```python
from build123d import *

# Parameters (mm, degrees)
SKETCH1_R           = 50.8
BOSS_EXTRUDE1_DEPTH = 203.2
SKETCH2_W           = 63.5
SKETCH2_H           = 79.31147458
BOSS_EXTRUDE2_DEPTH = 63.5
SKETCH3_W           = 25.4
SKETCH3_H           = 79.31147458
CUT_EXTRUDE1_DEPTH  = 63.5
FILLET1_R           = 25.4
SKETCH4_R           = 31.75
CUT_EXTRUDE2_DEPTH  = 63.5
SKETCH6_W           = 101.6
SKETCH6_H           = 101.6
BOSS_EXTRUDE3_DEPTH = 254
SKETCH7_W           = 106.066491774
SKETCH7_H           = 101.6
CUT_EXTRUDE4_DEPTH  = 409.182030472
CHAMFER2_SIZE       = 53.18
SKETCH5_R           = 12.7
BOSS_EXTRUDE5_DEPTH = 53.34
SKETCH11_R          = 38.1
CUT_EXTRUDE7_DEPTH  = 50.8


with BuildPart() as part:
    # Sketch1 → Boss-Extrude1 (new body)
    with BuildSketch(Plane(origin=(0, 0, 0), x_dir=(1, 0, 0), z_dir=(0, 1, 0))):
        with Locations(Location((0, 0, 0), (0, 0, 270))):
            Circle(SKETCH1_R)
    extrude(amount=BOSS_EXTRUDE1_DEPTH)

    # Sketch2 → Boss-Extrude2 (add)
    with BuildSketch(Plane(origin=(0, 203.2, 0), x_dir=(1, 0, 0), z_dir=(0, 1, 0))):
        Rectangle(SKETCH2_W, SKETCH2_H)
    extrude(amount=BOSS_EXTRUDE2_DEPTH)

    # Sketch3 → Cut-Extrude1 (cut)
    with BuildSketch(Plane(origin=(0, 266.7, 0), x_dir=(1, 0, 0), z_dir=(0, 1, 0))):
        Rectangle(SKETCH3_W, SKETCH3_H)
    extrude(amount=-CUT_EXTRUDE1_DEPTH, mode=Mode.SUBTRACT)

    # Fillet1
    fillet1_edges = [part.edges().sort_by_distance(p)[0] for p in [
        (22.225, 266.7, -39.65573729),
        (-22.225, 266.7, 39.65573729),
        (-22.225, 266.7, -39.65573729),
        (22.225, 266.7, 39.65573729),
    ]]
    fillet(fillet1_edges, radius=FILLET1_R)

    # Sketch4 → Cut-Extrude2 (cut)
    with BuildSketch(Plane.XZ):
        with Locations(Location((0, 0, 0), (0, 0, 270))):
            Circle(SKETCH4_R)
    extrude(amount=-CUT_EXTRUDE2_DEPTH, mode=Mode.SUBTRACT)

    # Sketch6 → Boss-Extrude3 (add)
    with BuildSketch(Plane.XY):
        with Locations((0, 152.4)):
            Rectangle(SKETCH6_W, SKETCH6_H)
    extrude(amount=BOSS_EXTRUDE3_DEPTH)

    # Sketch7 → Cut-Extrude4 (cut, through all)
    with BuildSketch(Plane.XY.offset(254)):
        with Locations((2.233245887, 50.8)):
            Rectangle(SKETCH7_W, SKETCH7_H)
    extrude(amount=-CUT_EXTRUDE4_DEPTH, mode=Mode.SUBTRACT)

    # Chamfer2
    chamfer2_edges = [part.edges().sort_by_distance(p)[0] for p in [
        (0, 203.2, 254),
    ]]
    chamfer(chamfer2_edges, length=CHAMFER2_SIZE)

    # Sketch5 → Boss-Extrude5 (add)
    with BuildSketch(Plane(origin=(31.75, 0, 0), x_dir=(0, 0, -1), z_dir=(1, 0, 0))):
        with Locations((0, 245.993497046)):
            Circle(SKETCH5_R)
    extrude(amount=-BOSS_EXTRUDE5_DEPTH)

    # Sketch11 → Cut-Extrude7 (cut)
    with BuildSketch(Plane.XZ.offset(-101.6)):
        with Locations(Location((0, 127, 0), (0, 0, 270))):
            Circle(SKETCH11_R)
    extrude(amount=-CUT_EXTRUDE7_DEPTH, mode=Mode.SUBTRACT)


solid = part.part
```
For this review, take the finished solid that the model builds, in its own axes (mm). A direction names the side the tool comes from. Round coordinates to 2 decimals unless told otherwise and drop trailing zeros. Write each loop counter-clockwise with the first axis right and the second up, starting at its lowest first coordinate (ties: lowest second). Pieces come first, ordered by that corner, then holes. Notation, with made-up numbers: (86, 75) - (107, 75) arc R17 ccw to (107, 96) - close; hole circle Ø1 at (46.25, 4.25). An arc over 180 degrees is marked (long way). Use CSV: the item, a comma, the result in double quotes.
1) For faces 4 (the flat face through (-12.7, 228, 1)), 5 (the flat face through (-22, 222, -39.656)), 6 (the flat face through (31.75, 235, 1)), list the 3-axis set-ups (+Z, -Z, +X, -X, +Y, -Y) from which the entire face can be reached by the end or side of a thin tool; tool diameter is ignored.
Conclusion:
face 4,"none"
face 5,"-Z, +X, -X, +Y"
face 6,"+Z, -Z, +X, +Y"
2) Clearance check with flat-ended pins moving along their axes: pin 1 Ø5 at (x, y) = (14, 183.5) entering from +Z; pin 2 Ø5.5 at (x, y) = (21.5, 230) entering from +Z; pin 3 Ø5.5 at (x, y) = (-19.5, 213) entering from -Z. State where each tip first meets the part, or that it passes through.
Conclusion:
pin 1,"stops at z = 223.02"
pin 2,"stops at z = 39.66"
pin 3,"stops at z = -39.66"
3) Wall thickness on line 1 along X through (y, z) = (129, 127); line 2 along X through (y, z) = (255, -30); line 3 along Y through (x, z) = (8.5, 188.5): over which ranges is each line inside the solid? List them lowest first. Write a range as from..to.
Conclusion:
line 1,"x = -50.8..-38.1, 38.1..50.8"
line 2,"x = -31.75..-12.7, 12.7..31.75"
line 3,"y = 101.6..203.2"
4) The part is to be moulded in two halves that separate along Z. For faces 1 (the flat face through (22, 222, -39.656)), 2 (the cylindrical face through (1.675, 126.644, 165.063)), 3 (the flat face through (-50.8, 152, 125)), say which applies: pulls with the +Z half, pulls with the -Z half, needs draft (parallel to the pull), parting line crosses it, or undercut.
Conclusion:
face 1,"pulls with the -Z half"
face 2,"undercut"
face 3,"needs draft"
5) Add section D-D on x = 43. Write out the cut boundary in (y, z).
Conclusion:
outline,"(101.6, -27.05) - (203.2, -27.05) - (203.2, 200.82) - (150.02, 254) - (101.6, 254) - close"
6) Add section B-B on x = 6.5. Write out the cut boundary in (y, z).
Conclusion:
outline,"(101.6, -50.38) - (203.2, -50.38) - (203.2, 200.82) - (150.02, 254) - (101.6, 254) - (101.6, 164.54) - (152.4, 164.54) - (152.4, 89.46) - (101.6, 89.46) - close; circle Ø25.4 at (245.99, 0)"
7) Add section A-A on y = 135. Write out the cut boundary in (x, z), and give its area (3 significant figures).
Conclusion:
outline,"(-50.8, 0) arc R50.8 ccw to (50.8, 0) - (50.8, 254) - (-50.8, 254) - close; hole circle Ø76.2 at (0, 127)"
area,"25,300 mm^2"
8) Add section C-C on z = 127. Write out the cut boundary in (x, y), and give its area (3 significant figures).
Conclusion:
outline,"(-50.8, 101.6) - (-38.1, 101.6) - (-38.1, 152.4) - (38.1, 152.4) - (38.1, 101.6) - (50.8, 101.6) - (50.8, 203.2) - (-50.8, 203.2) - close"
area,"6,450 mm^2"
